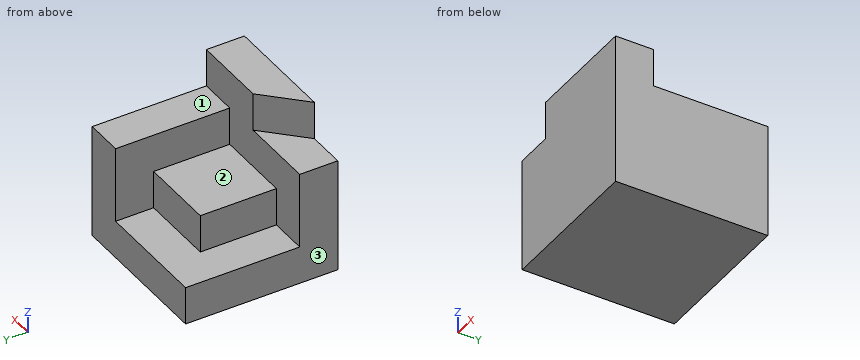
```python
from build123d import *

# Parameters (mm, degrees)
SKETCH1_W           = 40
SKETCH1_H           = 40
BOSS_EXTRUDE1_DEPTH = 40
SKETCH2_W           = 10
SKETCH2_H           = 10
CUT_EXTRUDE1_DEPTH  = 40
SKETCH4_W           = 10
SKETCH4_H           = 30
CUT_EXTRUDE3_DEPTH  = 40
CUT_EXTRUDE4_DEPTH  = 10
CUT_EXTRUDE5_DEPTH  = 30
SKETCH7_W           = 20
SKETCH7_H           = 10
CUT_EXTRUDE6_DEPTH  = 10


with BuildPart() as part:
    # Sketch1 → Boss-Extrude1 (new body)
    with BuildSketch(Plane.XY):
        with Locations((20, 20)):
            Rectangle(SKETCH1_W, SKETCH1_H)
    extrude(amount=BOSS_EXTRUDE1_DEPTH)

    # Sketch2 → Cut-Extrude1 (cut)
    with BuildSketch(Plane(origin=(0, 40, 0), x_dir=(1, 0, 0), z_dir=(0, 1, 0))):
        with Locations((5, -35)):
            Rectangle(SKETCH2_W, SKETCH2_H)
    extrude(amount=-CUT_EXTRUDE1_DEPTH, mode=Mode.SUBTRACT)

    # Sketch4 → Cut-Extrude3 (cut)
    with BuildSketch(Plane.ZY.offset(-10)):
        with Locations((35, 25)):
            Rectangle(SKETCH4_W, SKETCH4_H)
    extrude(amount=-CUT_EXTRUDE3_DEPTH, mode=Mode.SUBTRACT)

    # Sketch5 → Cut-Extrude4 (cut)
    with BuildSketch(Plane.XY.offset(40)):
        Polygon((10, 0), (20, 10), (10, 10), align=None)
    extrude(amount=-CUT_EXTRUDE4_DEPTH, mode=Mode.SUBTRACT)

    # Sketch6 → Cut-Extrude5 (cut)
    with BuildSketch(Plane(origin=(0, 40, 0), x_dir=(1, 0, 0), z_dir=(0, 1, 0))):
        Polygon((0, -30), (20, -30), (30, -30), (30, -20), (10, -20), (10, -10), (0, -10), align=None)
    extrude(amount=-CUT_EXTRUDE5_DEPTH, mode=Mode.SUBTRACT)

    # Sketch7 → Cut-Extrude6 (cut)
    with BuildSketch(Plane.XY.offset(20)):
        with Locations((20, 35)):
            Rectangle(SKETCH7_W, SKETCH7_H)
    extrude(amount=-CUT_EXTRUDE6_DEPTH, mode=Mode.SUBTRACT)


solid = part.part
```
Geometry check sheet. Reference: the model listing, model coordinates, mm. Face numbers are marked on the shaded views. A direction names the side the tool comes from. Coordinates: 2 decimals unless noted, no trailing zeros. Order: outer loops, then holes, each group sorted by start corner. A loop starts at its lowest first (then second) coordinate and runs counter-clockwise, first axis right, second up. Notation, with made-up numbers: M 29,28 L 84,28 A11 ccw 84,48 Z; hole C 29,-18.5 d6. An arc over 180 degrees is marked long. Answer as a JSON object with one key per item and string values.
Q1. Cross-section at C-C on x = 36. Record the cut outline in (y, z), and give its area (3 significant figures).
Results are:
{"outline": "M 0,0 L 40,0 L 40,30 L 10,30 L 10,40 L 0,40 Z", "area": "1,300 mm²"}
Q2. Cross-section at A-A on y = 16. Record the cut outline in (x, z), and give its area (3 significant figures).
Results are:
{"outline": "M 0,0 L 40,0 L 40,30 L 30,30 L 30,20 L 10,20 L 10,10 L 0,10 Z", "area": "800 mm²"}
Q3. Cross-section at B-B on z = 17. Record the cut outline in (x, y), and give its area (3 significant figures).
Results are:
{"outline": "M 0,0 L 40,0 L 40,40 L 30,40 L 30,30 L 10,30 L 10,10 L 0,10 Z", "area": "1,100 mm²"}
Q4. Depth check by flat-ended pin: pin 1 Ø6 at (y, z) = (21, 16) entering from -X; pin 2 Ø9 at (x, z) = (25, 22) entering from +Y; pin 3 Ø6 at (x, y) = (28.5, 31) entering from +Z. Enter the tip coordinate at first touch or a pass-through.
Results are:
{"pin 1": "stops at x = 10", "pin 2": "stops at y = 30", "pin 3": "stops at z = 30"}
Q5. Cross-section at D-D on z = 22.5. Record the cut outline in (x, y), and give its area (3 significant figures).
Results are:
{"outline": "M 0,0 L 40,0 L 40,40 L 30,40 L 30,10 L 0,10 Z", "area": "700 mm²"}
Q6. Scan lines: line 1 (Z direction, x = 37, y = 26); line 2 (X direction, y = 15.5, z = 25); line 3 (Z direction, x = 8.5, y = 24). Record each from-to range of solid material in increasing order.
Results are:
{"line 1": "z = 0 to 30", "line 2": "x = 30 to 40", "line 3": "z = 0 to 10"}
Q7. Tool access check on the marked faces 1, 2 and 3. Record the directions out of +Z, -Z, +X, -X, +Y, -Y that give a thin tool (end or side, any length) a straight path to the whole face; none if there is none.
Results are:
{"face 1": "+Z, +X, -X, +Y", "face 2": "+Z, -X, +Y", "face 3": "+Z, -Z, -X, +Y, -Y"}
